```python
from build123d import *

# Parameters (mm, degrees)
F0_R     = 7.5
F1_DEPTH = 6
F2_R     = 5.75
F3_DEPTH = 6
F4_R     = 2.5
F5_DEPTH = 6
F6_R     = 4.5
F7_DEPTH = 6
F8_R     = 1.5
F9_DEPTH = 25


with BuildPart() as f1:
    # F0 (on Top) → F1 (new body)
    with BuildSketch(Plane.XY):
        Circle(F0_R)
    extrude(amount=F1_DEPTH)

    # F2 (on face) → F3 (join)
    with BuildSketch(Plane.XY.offset(6)):
        Circle(F2_R)
    extrude(amount=F3_DEPTH)

    # F4 (on face) → F5 (cut)
    with BuildSketch(Plane.XY.offset(12)):
        Circle(F4_R)
    extrude(amount=-F5_DEPTH, mode=Mode.SUBTRACT)

    # F6 (on face) → F7 (cut)
    with BuildSketch(Plane(origin=(0, 0, 0), x_dir=(1, 0, 0), z_dir=(0, 0, -1))):
        Circle(F6_R)
    extrude(amount=-F7_DEPTH, mode=Mode.SUBTRACT)

    # F8 (on Right) → F9 (cut)
    with BuildSketch(Plane.YZ):
        with Locations((0, 3)):
            Circle(F8_R)
        with Locations((0, 9)):
            Circle(F8_R)
    extrude(amount=-F9_DEPTH, mode=Mode.SUBTRACT)


solid = f1.part
```
Here's how the part is built. I have some questions about the finished solid (model axes, mm). A direction names the side the tool comes from. Round coordinates to 2 decimals unless told otherwise and drop trailing zeros. Order: outer loops, then holes, each group sorted by start corner. A loop starts at its lowest first (then second) coordinate and runs counter-clockwise, first axis right, second up. Notation, with made-up numbers: (-26, 13.5) -> (-21, 13.5) arc R20 ccw to (-21, 52.5) -> close; hole circle Ø6 at (-14.5, 62). An arc over 180 degrees is marked (long way). Use a Markdown table: item, result. Add a question column.
(1) For pin 1 Ø2 at (x, z) = (-2.5, 5.5) entering from -Y; pin 2 Ø3 at (x, y) = (0, 0) entering from -Z; pin 3 Ø4 at (x, z) = (-2.5, 10) entering from -Y; pin 4 Ø2.5 at (x, y) = (2, -1.5) entering from -Z, each with a flat end and sliding along its axis, tell me the tip position at first contact or that it passes through.
(2) If we mould it in two halves opening along Y, with no side actions, what happens to faces 1 (the face through (-5.85, -1.5, 3.07)), 2 (the face through (-2, -6, 6)), 3 (the face through (5.484, 1.727, 8.958))? For each: released by +Y, released by -Y, zero draft, split by the parting line, or undercut.
(3) I need wall thicknesses on line 1 along Y through (x, z) = (0, 4.5); line 2 along Y through (x, z) = (0, 10); line 3 along Z through (x, y) = (5.5, -3). Which ranges of each line are inside material? Lowest first, please.
(4) Suppose I cut it at A-A, the plane x = 0. Please give me the cut outline in (y, z), and give its area (3 significant figures).
(5) Suppose I cut it at D-D, the plane x = -6. Please give me the cut outline in (y, z), and give its area (3 significant figures).
(6) For faces 4 (the face through (0, -5, 0)), 5 (the face through (-3.851, 1.386, 8.425)), 6 (the face through (4.292, -1.352, 2.958)), which set-ups out of +Z, -Z, +X, -X, +Y, -Y let a thin tool reach every point of the face, with its end or its side?
(7) Suppose I cut it at C-C, the plane z = 11.25. Please give me the cut outline in (x, y).
(8) Suppose I cut it at B-B, the plane y = 0. Please give me the cut outline in (x, z).
Verdict:
| question | item | result |
|---|---|---|
| 1 | pin 1 | y = -7.35 |
| 1 | pin 2 | through |
| 1 | pin 3 | y = -5.73 |
| 1 | pin 4 | z = 6 |
| 2 | face 1 | undercut |
| 2 | face 2 | zero draft |
| 2 | face 3 | split by the parting line |
| 3 | line 1 | -7.5 to -4.5, 4.5 to 7.5 |
| 3 | line 2 | -5.75 to -2.5, 2.5 to 5.75 |
| 3 | line 3 | 0 to 6 |
| 4 | outline | (-7.5, 0) -> (-4.5, 0) -> (-4.5, 6) -> (-2.5, 6) -> (-2.5, 12) -> (-5.75, 12) -> (-5.75, 6) -> (-7.5, 6) -> close; (2.5, 6) -> (4.5, 6) -> (4.5, 0) -> (7.5, 0) -> (7.5, 6) -> (5.75, 6) -> (5.75, 12) -> (2.5, 12) -> close |
| 4 | area | 75.0 mm2 |
| 5 | outline | (-4.5, 0) -> (4.5, 0) -> (4.5, 6) -> (-4.5, 6) -> close; hole circle Ø3 at (0, 3) |
| 5 | area | 46.9 mm2 |
| 6 | face 4 | -Z, +X, -X, +Y, -Y |
| 6 | face 5 | -X |
| 6 | face 6 | -Z |
| 7 | outline | circle Ø11.5 at (0, 0); hole circle Ø5 at (0, 0) |
| 8 | outline | (-7.5, 0) -> (-4.5, 0) -> (-4.5, 1.5) -> (-7.5, 1.5) -> close; (-7.5, 4.5) -> (-4.5, 4.5) -> (-4.5, 6) -> (-2.5, 6) -> (-2.5, 7.5) -> (-5.75, 7.5) -> (-5.75, 6) -> (-7.5, 6) -> close; (-5.75, 10.5) -> (-2.5, 10.5) -> (-2.5, 12) -> (-5.75, 12) -> close; (2.5, 6) -> (4.5, 6) -> (4.5, 0) -> (7.5, 0) -> (7.5, 6) -> (5.75, 6) -> (5.75, 12) -> (2.5, 12) -> close |
